Work out the finished part from the listing and answer in its coordinate system (mm). Face numbers are marked on the shaded views. A direction names the side the tool comes from. Coordinates: 2 decimals unless noted, no trailing zeros. Loops run counter-clockwise (first coordinate to the right, second up) from the corner with the lowest first, then second, coordinate; pieces in that order, holes last. Notation, with made-up numbers: (66.25, 18) - (75.25, 18) arc R13 cw to (75.25, 25) - close; hole circle Ø3 at (-26, 75). An arc over 180 degrees is marked (long way). Write each question's results on one line, items separated by ' | '. Start each with the question number.
Item 1: Section B-B, the plane y = -25 is taken. Write down the section's boundary in (x, z), plus the area to 3 significant figures.
Item 2: Consider probe 1 along Y at (x, z) = (-17.5, 2); probe 2 along Z at (x, y) = (2.5, -27.5); probe 3 along X at (y, z) = (-25, -5). Determine where each line is inside the solid, lowest interval first. Write a range as [from, to].
Item 3: A tool of negligible diameter and unlimited length cuts with its end or side. For the marked faces 1, 2, 3, 4 and 5, from which of +Z, -Z, +X, -X, +Y, -Y can it reach the whole face along a straight path? Write none if from no direction.
Item 4: Section A-A, the plane y = -15 is taken. Write down the section's boundary in (x, z).
Item 5: This flat-tipped pin is pushed along its axis until it touches: pin 1 Ø1.3 at (x, y) = (17.5, -25) entering from +Z. Where does it stop, or does it pass through?
Item 6: Section D-D, the plane x = -17.5 is taken. Write down the section's boundary in (y, z), plus the area to 3 significant figures.
Item 7: For a pull along Y with two mould halves and no side action, classify the marked faces 6, 7 and 8 as +Y half, -Y half, draft (parallel to the pull), parting line (faces both ways), or undercut.
Item 8: Section C-C, the plane x = -12 is taken. Write down the section's boundary in (y, z).
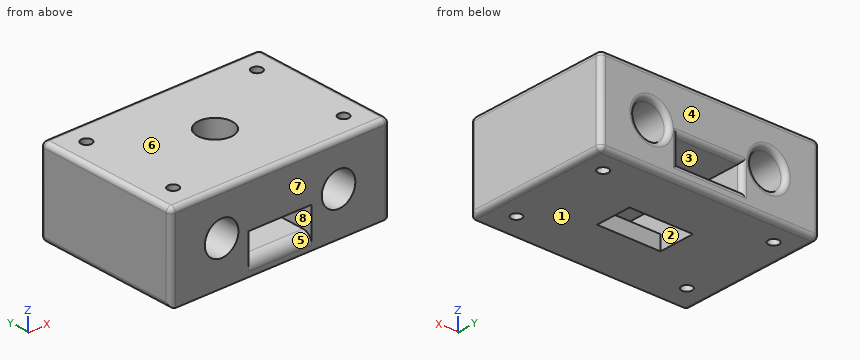
from build123d import *

# Parameters (mm, degrees)
SKETCH_W        = 45
SKETCH_H        = 17.5
SKETCH_R        = 3.45
SKETCH_W_2      = 13
SKETCH_H_2      = 5
PAD_DEPTH       = 30
SKETCH001_R     = 3.55
SKETCH001_R_2   = 1.075196
SKETCH001_R_3   = 1.087844
POCKET_DEPTH    = 131.18917
SKETCH002_W     = 13
SKETCH002_H     = 7.5
POCKET001_DEPTH = 5
FILLET_R        = 1
FILLET001_R     = 2


with BuildPart() as part:
    # Sketch → Pad (new body)
    with BuildSketch(Plane.XZ):
        Rectangle(SKETCH_W, SKETCH_H)
        with Locations((-12, 0)):
            Circle(SKETCH_R, mode=Mode.SUBTRACT)
        with Locations((12, 0)):
            Circle(SKETCH_R, mode=Mode.SUBTRACT)
        with Locations((0, -3.25)):
            Rectangle(SKETCH_W_2, SKETCH_H_2, mode=Mode.SUBTRACT)
    extrude(amount=PAD_DEPTH)

    # Sketch001 (on DatumPlane) → Pocket (cut, through all)
    with BuildSketch(Plane(origin=(0, 0, 8.75), x_dir=(-1, 0, 0), z_dir=(0, 0, 1))):
        with Locations((0, 15)):
            Circle(SKETCH001_R)
        with Locations((17.5, 25)):
            Circle(SKETCH001_R_2)
        with Locations((17.5, 5)):
            Circle(SKETCH001_R_3)
    pocket = extrude(amount=-POCKET_DEPTH, mode=Mode.SUBTRACT)

    # Mirrored: Pocket across Sketch001 V_Axis
    add(pocket.mirror(Plane(origin=(0, 0, 8.75), x_dir=(0, 0, 1), z_dir=(-1, 0, 0))), mode=Mode.SUBTRACT)

    # Sketch002 (on Face1 of Mirrored) → Pocket001 (cut)
    with BuildSketch(Plane(origin=(0, 0, -8.75), x_dir=(1, 0, 0), z_dir=(0, 0, -1))):
        with Locations((0, 15)):
            Rectangle(SKETCH002_W, SKETCH002_H)
    extrude(amount=-POCKET001_DEPTH, mode=Mode.SUBTRACT)

    # Fillet
    fillet_edges = [part.edges().sort_by_distance(p)[0] for p in [
        (-22.5, -15, 8.75),
        (-22.5, -15, -8.75),
        (-22.5, 0, 0),
        (-22.5, -30, 0),
        (22.5, -15, -8.75),
        (22.5, -15, 8.75),
        (22.5, 0, 0),
        (22.5, -30, 0),
        (0, 0, -8.75),
        (0, 0, 8.75),
        (0, 0, -5.75),
        (6.5, 0, -3.25),
        (0, 0, -0.75),
        (-6.5, 0, -3.25),
        (8.55, 0, 0),
        (-15.45, 0, 0),
        (0, -30, 8.75),
    ]]
    fillet(fillet_edges, radius=FILLET_R)

    # Fillet001
    fillet001_edges = [part.edges().sort_by_distance(p)[0] for p in [
        (0, -30, -5.75),
    ]]
    fillet(fillet001_edges, radius=FILLET001_R)


solid = part.part
Answer key:
1) outline: (-22.5, -7.75) arc R1 ccw to (-21.5, -8.75) - (-18.58, -8.75) - (-18.58, 8.75) - (-21.5, 8.75) arc R1 ccw to (-22.5, 7.75) - close; (-16.42, -8.75) - (16.42, -8.75) - (16.42, 8.75) - (-16.42, 8.75) - close; (18.58, -8.75) - (21.5, -8.75) arc R1 ccw to (22.5, -7.75) - (22.5, 7.75) arc R1 ccw to (21.5, 8.75) - (18.58, 8.75) - close; hole circle Ø6.9 at (-12, 0); hole (-6.5, -5.75) - (6.5, -5.75) - (6.5, -0.75) - (-6.5, -0.75) - close; hole circle Ø6.9 at (12, 0) | area: 572 mm^2
2) probe 1: y = [-30, -26.08], [-23.92, -6.09], [-3.91, 0] | probe 2: z = [-8.75, -5.75], [-0.75, 8.75] | probe 3: x = [-22.5, -18.58], [-16.42, -6.5], [6.5, 16.42], [18.58, 22.5]
3) face 1: -Z, +X, -X, +Y, -Y | face 2: none | face 3: +Y, -Y | face 4: +Z, -Z, +X, -X, +Y | face 5: -Y
4) outline: (-22.5, -7.75) arc R1 ccw to (-21.5, -8.75) - (-6.5, -8.75) - (-6.5, -0.75) - (-3.55, -0.75) - (-3.55, 8.75) - (-21.5, 8.75) arc R1 ccw to (-22.5, 7.75) - close; (3.55, -0.75) - (6.5, -0.75) - (6.5, -8.75) - (21.5, -8.75) arc R1 ccw to (22.5, -7.75) - (22.5, 7.75) arc R1 ccw to (21.5, 8.75) - (3.55, 8.75) - close; hole circle Ø6.9 at (-12, 0); hole circle Ø6.9 at (12, 0)
5) pin 1: passes through
6) outline: (-30, -8.75) - (-26.08, -8.75) - (-26.08, 8.75) - (-29, 8.75) arc R1 ccw to (-30, 7.75) - close; (-23.92, -8.75) - (-6.09, -8.75) - (-6.09, 8.75) - (-23.92, 8.75) - close; (-3.91, -8.75) - (-1, -8.75) arc R1 ccw to (0, -7.75) - (0, 7.75) arc R1 ccw to (-1, 8.75) - (-3.91, 8.75) - close | area: 449 mm^2
7) face 6: draft | face 7: -Y half | face 8: undercut
8) outline: (-30, -8.75) - (-1, -8.75) arc R1 ccw to (0, -7.75) - (0, -4.45) arc R1 ccw to (-1, -3.45) - (-30, -3.45) - close; (-30, 3.45) - (-1, 3.45) arc R1 ccw to (0, 4.45) - (0, 7.75) arc R1 ccw to (-1, 8.75) - (-29, 8.75) arc R1 ccw to (-30, 7.75) - close
